Here's the drawing with two shaded views (mm, measured from the low corner). I have some questions. A direction names the side the tool comes from. Round coordinates to 2 decimals unless told otherwise and drop trailing zeros. Loops run counter-clockwise (first coordinate to the right, second up) from the corner with the lowest first, then second, coordinate; pieces in that order, holes last. Notation, with made-up numbers: (53.5, 52) - (99.5, 52) arc R23 ccw to (99.5, 67) - close; hole circle Ø8 at (-7, -29.75). An arc over 180 degrees is marked (long way). Answer as CSV lines item,"result".
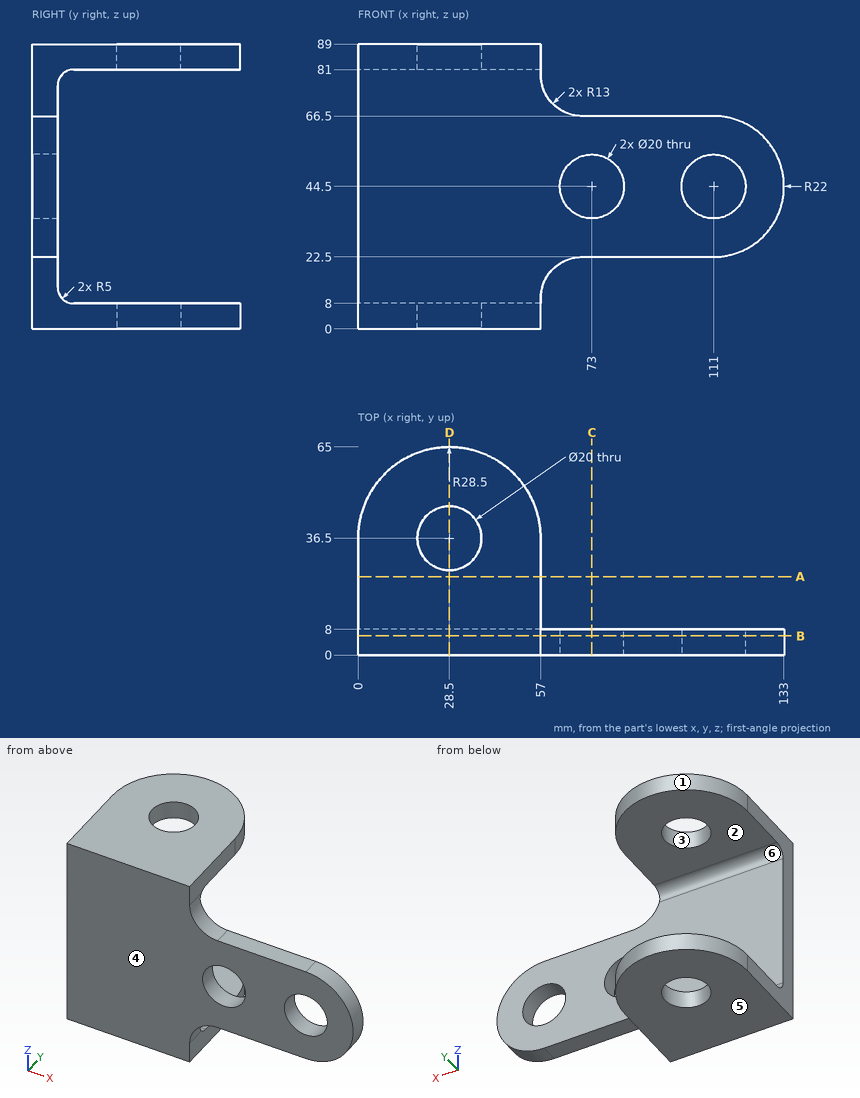
Q1. Imagine slicing it at D-D (x = 28.5). Write out the boundary of the cut face in (y, z).
Checks:
outline,"(0, 0) - (26.5, 0) - (26.5, 8) - (13, 8) arc R5 cw to (8, 13) - (8, 76) arc R5 cw to (13, 81) - (26.5, 81) - (26.5, 89) - (0, 89) - close; (46.5, 0) - (65, 0) - (65, 8) - (46.5, 8) - close; (46.5, 81) - (65, 81) - (65, 89) - (46.5, 89) - close"
Q2. We'd pull the mould along Y, two halves only. Please class the marked faces 1, 2, 3 and 4: pulls with the +Y half, pulls with the -Y half, needs draft (parallel to the pull), parting line crosses it, or undercut.
Checks:
face 1,"pulls with the +Y half"
face 2,"needs draft"
face 3,"undercut"
face 4,"pulls with the -Y half"
Q3. If I drill on line 1 along X through (y, z) = (3, 44); line 2 along Y through (x, z) = (28, 87); line 3 along Z through (x, y) = (38.5, 46.5), over which ranges is the centre line in solid material (lowest first)? Write a range as [from, to].
Checks:
line 1,"[0, 63.01], [82.99, 101.01], [120.99, 132.99]"
line 2,"[0, 26.51], [46.49, 65]"
line 3,"[0, 8], [81, 89]"
Q4. Imagine slicing it at C-C (x = 73). Write out the boundary of the cut face in (y, z).
Checks:
outline,"(0, 22.5) - (8, 22.5) - (8, 34.5) - (0, 34.5) - close; (0, 54.5) - (8, 54.5) - (8, 66.5) - (0, 66.5) - close"
Q5. On a 3-axis mill with a long thin cutter (end or side, diameter ignored), from which of +Z, -Z, +X, -X, +Y, -Y can I reach the whole of each face in a straight line? I mean the marked faces 5 and 6. Say none if no direction works.
Checks:
face 5,"-Z, +X, -X, +Y, -Y"
face 6,"+X, -X, +Y"
Q6. Imagine slicing it at B-B (y = 6). Write out the boundary of the cut face in (x, z), then the cut area to 3 significant figures.
Checks:
outline,"(0, 0) - (57, 0) - (57, 9.5) arc R13 cw to (70, 22.5) - (111, 22.5) arc R22 ccw to (111, 66.5) - (70, 66.5) arc R13 cw to (57, 79.5) - (57, 89) - (0, 89) - close; hole circle Ø20 at (73, 44.5); hole circle Ø20 at (111, 44.5)"
area,"7,650 mm²"
Q7. I'm going to push flat-ended pins straight in: pin 1 Ø18 at (x, y) = (28.5, 36.5) entering from -Z; pin 2 Ø6.5 at (x, y) = (82.5, 4.5) entering from -Z; pin 3 Ø1 at (x, y) = (18, 24.5) entering from -Z; pin 4 Ø10.5 at (y, z) = (26.5, 83) entering from +X. Where does each tip first touch, or does it pass through?
Checks:
pin 1,"through"
pin 2,"z = 22.5"
pin 3,"z = 0"
pin 4,"x = 57"
Q8. Imagine slicing it at A-A (y = 24.5). Write out the boundary of the cut face in (x, z), then the cut area to 3 significant figures.
Checks:
outline,"(0, 0) - (57, 0) - (57, 8) - (0, 8) - close; (0, 81) - (57, 81) - (57, 89) - (0, 89) - close"
area,"912 mm²"
